Geometry: final body of the model. Coordinates: model frame, mm. Face numbers are marked on the shaded views. Round coordinates to 2 decimals unless told otherwise and drop trailing zeros. Write each loop counter-clockwise with the first axis right and the second up, starting at its lowest first coordinate (ties: lowest second). Pieces come first, ordered by that corner, then holes. Notation, with made-up numbers: M -14,-33 L 27,-33 A24 cw 27,-1 Z; hole C -6.5,2 d8. An arc over 180 degrees is marked long. Use one line per item in the form item = value. Start each with the question number.
Item 1: Ray query, probe 1 along Z at (x, y) = (0, 0); probe 2 along Y at (x, z) = (0, 2.25); probe 3 along Y at (x, z) = (-0.75, 0.5). Return the intervals inside material, ascending.
Item 2: Pull-direction query (Y, two-part tool) for the marked faces 1, 2 and 3; classes: pulls with the +Y half, pulls with the -Y half, needs draft (parallel to the pull), parting line crosses it, or undercut.
Item 3: Section query C-C (y = 0). Return loops of the section in (x, z).
Item 4: Section query B-B (x = 0.5). Return loops of the section in (y, z), and give its area (3 significant figures).
Item 5: Pin query (flat end, axial travel): pin 1 Ø3 at (x, z) = (-1, -4.5) entering from +Y. Return the tip coordinate at first contact, or that it passes through.
Item 6: Section query A-A (z = 0). Return loops of the section in (x, y).
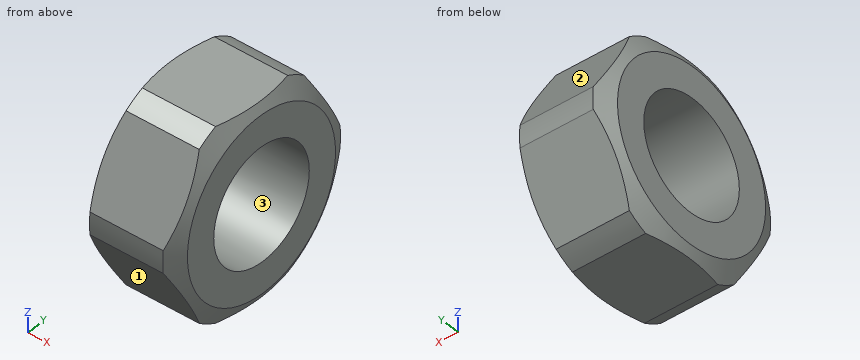
from build123d import *

# Parameters (mm, degrees)
SKETCH_2_OUTSIDE_W  = 26.122
SKETCH_2_OUTSIDE_H  = 26.122
CUT_EXTRUDE_1_DEPTH = 9.4


with BuildPart() as part:
    # Эскиз1 → Повернуть1 (revolve)
    with BuildSketch(Plane.XY):
        Polygon((4.2, 5), (-4.2, 5), (-4.2, 7.75), (-3.305107083, 9.3), (3.305107083, 9.3), (4.2, 7.75), align=None)
    revolve(axis=Axis((-345.378129483, 0, 0), (1, 0, 0)))

    # Эскиз2 outside → Вырез-Вытянуть1 (cut, through all)
    with BuildSketch(Plane.ZY.offset(4.2)):
        Rectangle(SKETCH_2_OUTSIDE_W, SKETCH_2_OUTSIDE_H)
        Polygon((0, -9.814954576), (8.5, -4.907477288), (8.5, 4.907477288), (0, 9.814954576), (-8.5, 4.907477288), (-8.5, -4.907477288), align=None, mode=Mode.SUBTRACT)
    extrude(amount=-CUT_EXTRUDE_1_DEPTH, mode=Mode.SUBTRACT)


solid = part.part
Working result:
q1.probe_1 = -8.5 to -5, 5 to 8.5
q1.probe_2 = -8.52 to -4.47, 4.47 to 8.52
q1.probe_3 = -9.29 to -4.97, 4.97 to 9.29
q2.face_1 = pulls with the -Y half
q2.face_2 = pulls with the +Y half
q2.face_3 = undercut
q3.outline = M -4.2,-7.75 L -3.77,-8.5 L 3.77,-8.5 L 4.2,-7.75 L 4.2,-5 L -4.2,-5 Z; M -4.2,5 L 4.2,5 L 4.2,7.75 L 3.77,8.5 L -3.77,8.5 L -4.2,7.75 Z
q4.outline = M -9.25,-0.98 L -5.47,-7.52 A9.3 ccw -3.77,-8.5 L 3.77,-8.5 A9.3 ccw 5.47,-7.52 L 9.25,-0.98 A9.3 ccw 9.25,0.98 L 5.47,7.52 A9.3 ccw 3.77,8.5 L -3.77,8.5 A9.3 ccw -5.47,7.52 L -9.25,0.98 A9.3 ccw Z; hole C 0,0 d10
q4.area = 169 mm²
q5.pin_1 = 8.08
q6.outline = M -4.2,-7.75 L -3.31,-9.3 L 3.31,-9.3 L 4.2,-7.75 L 4.2,-5 L -4.2,-5 Z; M -4.2,5 L 4.2,5 L 4.2,7.75 L 3.31,9.3 L -3.31,9.3 L -4.2,7.75 Z
